For this review, take the finished solid that the model builds, in its own axes (mm). A direction names the side the tool comes from. Coordinates: 2 decimals unless noted, no trailing zeros. Loops run counter-clockwise (first coordinate to the right, second up) from the corner with the lowest first, then second, coordinate; pieces in that order, holes last. Notation, with made-up numbers: M 41.5,-11 L 97.5,-11 A29 cw 97.5,13 Z; hole C 4.5,33.5 d9. An arc over 180 degrees is marked long. Use one line per item in the form item = value.
```python
from build123d import *

# Parameters (mm, degrees)
SKETCH1_W           = 76.2
SKETCH1_H           = 25.4
SKETCH1_W_2         = 69.85
SKETCH1_H_2         = 19.05
EXTRUDE_THIN1_DEPTH = 266.7
SKETCH2_R           = 2.032
CUT_EXTRUDE1_DEPTH  = 26.4


with BuildPart() as part:
    # Sketch1 → Extrude-Thin1 (new body, symmetric)
    with BuildSketch(Plane.XY):
        Rectangle(SKETCH1_W, SKETCH1_H)
        Rectangle(SKETCH1_W_2, SKETCH1_H_2, mode=Mode.SUBTRACT)
    extrude(amount=EXTRUDE_THIN1_DEPTH, both=True)

    # Sketch2 → Cut-Extrude1 (cut, through all)
    with BuildSketch(Plane(origin=(0, 12.7, 0), x_dir=(1, 0, 0), z_dir=(0, 1, 0))):
        with Locations((25.4, 254)):
            Circle(SKETCH2_R)
        with Locations((0, 254)):
            Circle(SKETCH2_R)
        with Locations((25.4, -254)):
            Circle(SKETCH2_R)
        with Locations((0, -254)):
            Circle(SKETCH2_R)
        with Locations((-25.4, 254)):
            Circle(SKETCH2_R)
        with Locations((-25.4, -254)):
            Circle(SKETCH2_R)
    extrude(amount=-CUT_EXTRUDE1_DEPTH, mode=Mode.SUBTRACT)


solid = part.part
```
1. Draft analysis for pull direction Y (two halves, no side actions). For faces 3 (the face through (0, -9.525, 4)), 4 (the face through (-1, 12.7, 4)), 5 (the face through (-3, -10, -266.7)), 6 (the face through (-1, -12.7, 4)), state which applies: +Y half, -Y half, draft (parallel to the pull), parting line (faces both ways), or undercut.
Computed values:
face_3 = undercut
face_4 = +Y half
face_5 = draft
face_6 = -Y half
2. Consider section A-A on y = 2. Write out the cut boundary in (x, z) (3 decimals), plus the area to 3 significant figures.
Computed values:
outline = M -38.1,-266.7 L -34.925,-266.7 L -34.925,266.7 L -38.1,266.7 Z; M 34.925,-266.7 L 38.1,-266.7 L 38.1,266.7 L 34.925,266.7 Z
area = 3,390 mm2
3. Wall thickness on line 1 along Z through (x, y) = (0, -11.75); line 2 along X through (y, z) = (10.95, 254); line 3 along Y through (x, z) = (-28, 215) (3 decimals): over which ranges is each line inside the solid? List them lowest first. Write a range as from..to.
Computed values:
line_1 = -266.7..-256.03, -251.97..251.97, 256.03..266.7
line_2 = -38.1..-27.43, -23.37..-2.03, 2.03..23.37, 27.43..38.1
line_3 = -12.7..-9.525, 9.525..12.7
4. Consider section B-B on x = 7.5. Write out the cut boundary in (y, z) (3 decimals).
Computed values:
outline = M -12.7,-266.7 L -9.525,-266.7 L -9.525,266.7 L -12.7,266.7 Z; M 9.525,-266.7 L 12.7,-266.7 L 12.7,266.7 L 9.525,266.7 Z
5. Tool access review of faces 1 (the face through (-3, -10, 266.7)), 2 (the face through (0, 9.525, 4)): name each direction out of +Z, -Z, +X, -X, +Y, -Y from which nothing blocks a thin tool from reaching the whole face with its end or side.
Computed values:
face_1 = +Z, +X, -X, +Y, -Y
face_2 = +Z, -Z
6. Consider section C-C on z = 154. Write out the cut boundary in (x, y) (3 decimals).
Computed values:
outline = M -38.1,-12.7 L 38.1,-12.7 L 38.1,12.7 L -38.1,12.7 Z; hole M -34.925,-9.525 L 34.925,-9.525 L 34.925,9.525 L -34.925,9.525 Z
